Check sheet for the modelled part. Datum: model origin and axes. Units: mm. Give positions to 0.01 mm unless a question says otherwise; leave off trailing zeros. Order: outer loops, then holes, each group sorted by start corner. A loop starts at its lowest first (then second) coordinate and runs counter-clockwise, first axis right, second up. Notation, with made-up numbers: (66, 65) -> (99, 65) arc R19 ccw to (99, 76) -> close; hole circle Ø6 at (-22.5, 23). An arc over 180 degrees is marked (long way). Answer in a Markdown table with one row per item. Add a question column.
(1) Go/stop test with a flat-tipped pin: pin 1 (7 mm diameter, centred on x = 18, z = -160, fed in from -Y). Record where the tip stops, or that it passes through.
(2) Cross-section at C-C (z = 50.5). Record the cut outline in (x, y), then the cut area to 3 significant figures.
(3) Cross-section at B-B (z = -160). Record the cut outline in (x, y).
(4) Thickness scan on L1, parallel to Z at x = 18, y = 2.8; L2, parallel to X at y = 3.95, z = -160; L3, parallel to Z at x = 87, y = 3.9. Record the ranges inside material, lowest first. Write a range as [from, to].
(5) Cross-section at A-A (x = 18). Record the cut outline in (y, z), then the cut area to 3 significant figures.
```python
from build123d import *

# Parameters (mm, degrees)
SKIZZE10_W                      = 100
SKIZZE10_H                      = 334
AUFSATZ_LINEAR_AUSTRAGEN1_DEPTH = 5
FASE1_SIZE                      = 4
DURCHGANGSLOCH_F_R_M81_D        = 9


with BuildPart() as part:
    # Skizze10 → Aufsatz-Linear austragen1 (new body)
    with BuildSketch(Plane(origin=(0, 0, 0), x_dir=(1, 0, 0), z_dir=(0, 1, 0))):
        with Locations((50, 0)):
            Rectangle(SKIZZE10_W, SKIZZE10_H)
    extrude(amount=AUFSATZ_LINEAR_AUSTRAGEN1_DEPTH)

    # Fase1
    fase1_edges = [part.edges().sort_by_distance(p)[0] for p in [
        (0, 0, 0),
    ]]
    chamfer(fase1_edges, length=FASE1_SIZE)

    # Durchgangsloch für M81 (through all)
    with Locations(Plane(origin=(0, 5, 0), x_dir=(1, 0, 0), z_dir=(0, 1, 0))):
        with Locations((18, -160), (18, 160), (88, -160), (88, 160)):
            Hole(DURCHGANGSLOCH_F_R_M81_D / 2)


solid = part.part
```
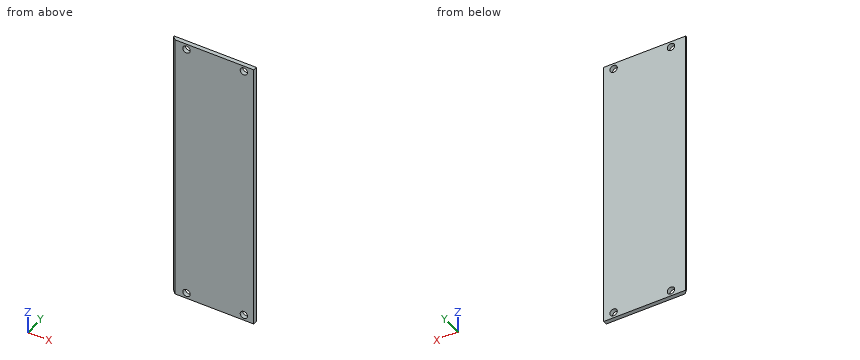
Answer below:
| question | item | result |
|---|---|---|
| 1 | pin 1 | passes through |
| 2 | outline | (0, 4) -> (4, 0) -> (100, 0) -> (100, 5) -> (0, 5) -> close |
| 2 | area | 492 mm² |
| 3 | outline | (0, 4) -> (4, 0) -> (13.5, 0) -> (13.5, 5) -> (0, 5) -> close; (22.5, 0) -> (83.5, 0) -> (83.5, 5) -> (22.5, 5) -> close; (92.5, 0) -> (100, 0) -> (100, 5) -> (92.5, 5) -> close |
| 4 | L1 | z = [-167, -164.5], [-155.5, 155.5], [164.5, 167] |
| 4 | L2 | x = [0.05, 13.5], [22.5, 83.5], [92.5, 100] |
| 4 | L3 | z = [-167, -164.39], [-155.61, 155.61], [164.39, 167] |
| 5 | outline | (0, -167) -> (5, -167) -> (5, -164.5) -> (0, -164.5) -> close; (0, -155.5) -> (5, -155.5) -> (5, 155.5) -> (0, 155.5) -> close; (0, 164.5) -> (5, 164.5) -> (5, 167) -> (0, 167) -> close |
| 5 | area | 1,580 mm² |
